Autodesk Inventor part; units mm, degrees
ref_plane "YZ Plane" through (0, 0, 0) normal (1, 0, 0) x (0, 1, 0)
ref_plane "XZ Plane" through (0, 0, 0) normal (0, 1, 0) x (-1, 0, 0)
ref_plane "XY Plane" through (0, 0, 0) normal (0, 0, 1) x (1, 0, 0)
sketch "Esquisse11" plane through (0, 0, 0) normal (1, 0, 0) x (0, 1, 0)
  line L0 (0, 0) -> (25, 0)
  line L1 (25, 0) -> (25, 10)
  line L2 (25, 10) -> (0, 10)
  line L3 (0, 10) -> (0, 0)
  line L4 (12.5, 0) -> (12.5, 10) construction
  circle A0 centre (12.5, 5) radius 2.15
  line L5 (12.5, 5) -> (25, 5) construction
  circle A1 centre (18.5, 5) radius 2.15
  circle A2 centre (6.5, 5) radius 2.15
  circle A3 centre (12.5, 5) radius 2.15
  dimension "d118" = 25
  dimension "d119" = 10
  dimension "d120" = 5
  dimension "d121" = 4.3
  dimension "d124" = 6
  dimension "d127" = 6
extrude "Extrusion11" add sketch "Esquisse11" along normal blind 2.2
fillet "Congé7" radius 7 2 edges at (1.1, 0, 0) (1.1, 25, 0)
mirror "Symétrie2" about plane through (0, 25, 10) normal (0, 0, 1)
equation "\"d121\" = Holes"
equation "\"d130\" = Depth"
equation "\"d132\" = Rounding"
equation "\"Depth\" = 2.2"
equation "\"Holes\" = 4.3"
equation "\"Height\" = 0"
equation "\"Rounding\" = 7"
properties part number "BottomToBottom"
Can you work these out from the model? Positions are in its coordinate system, mm. Coordinates: 2 decimals unless noted, no trailing zeros. Write each loop counter-clockwise with the first axis right and the second up, starting at its lowest first coordinate (ties: lowest second). Pieces come first, ordered by that corner, then holes. Notation, with made-up numbers: M -3.5,21.25 L 19.5,21.25 A15 ccw 19.5,43.25 Z; hole C 77.25,47 d2. An arc over 180 degrees is marked long. Write item = value, one per line. Start each with the question number.
Q1. If we section it at D-D, the plane y = 19.5: Write out the boundary of the cut face in (x, z).
Q2. I'm going to push a flat-ended pin straight in: pin 1 (1 mm diameter, centred on x = 1, y = 6, fed in from -Z). Where does the tip first touch, or does it pass through?
Q3. If I drill on L1, parallel to Z at x = 0.85, y = 12.5; L2, parallel to Y at x = 1.05, z = 5.25; L3, parallel to Z at x = 1.75, y = 19, over which ranges is the centre line in solid material (lowest first)? Write a range as [from, to].
Q4. If we section it at C-C, the plane z = 6: Write out the boundary of the cut face in (x, y).
Q5. Thinking about a two-plate mould opening in Z: for faces 1 (the face through (1, 13, 20)), 2 (the face through (1, 0, 10)), 3 (the face through (1.08, 19.49, 6.91)), which applies, released by +Z, released by -Z, zero draft, split by the parting line, or undercut?
Q6. If we section it at A-A, the plane y = 12.5: Write out the boundary of the cut face in (x, z).
Q7. If we section it at B-B, the plane x = 0.85: Write out the boundary of the cut face in (y, z).
Check sheet entries:
q1.outline = M 0,0.16 L 2.2,0.16 L 2.2,3.1 L 0,3.1 Z; M 0,6.9 L 2.2,6.9 L 2.2,13.1 L 0,13.1 Z; M 0,16.9 L 2.2,16.9 L 2.2,19.84 L 0,19.84 Z
q2.pin_1 = 0.02
q3.L1 = [0, 2.85], [7.15, 12.85], [17.15, 20]
q3.L2 = [0.22, 4.36], [8.64, 10.36], [14.64, 16.36], [20.64, 24.78]
q3.L3 = [0.07, 2.91], [7.09, 12.91], [17.09, 19.93]
q4.outline = M 0,0.07 L 2.2,0.07 L 2.2,4.6 L 0,4.6 Z; M 0,8.4 L 2.2,8.4 L 2.2,10.6 L 0,10.6 Z; M 0,14.4 L 2.2,14.4 L 2.2,16.6 L 0,16.6 Z; M 0,20.4 L 2.2,20.4 L 2.2,24.93 L 0,24.93 Z
q5.face_1 = released by +Z
q5.face_2 = zero draft
q5.face_3 = undercut
q6.outline = M 0,0 L 2.2,0 L 2.2,2.85 L 0,2.85 Z; M 0,7.15 L 2.2,7.15 L 2.2,12.85 L 0,12.85 Z; M 0,17.15 L 2.2,17.15 L 2.2,20 L 0,20 Z
q7.outline = M 0,7 A7 ccw 7,0 L 18,0 A7 ccw 25,7 L 25,13 A7 ccw 18,20 L 7,20 A7 ccw 0,13 Z; hole C 6.5,5 d4.3; hole C 6.5,15 d4.3; hole C 12.5,5 d4.3; hole C 12.5,15 d4.3; hole C 18.5,5 d4.3; hole C 18.5,15 d4.3
